Geometry: final body of the model. Coordinates: model frame, mm. Face numbers are marked on the shaded views. A direction names the side the tool comes from. Give positions to 0.01 mm unless a question says otherwise; leave off trailing zeros. Write each loop counter-clockwise with the first axis right and the second up, starting at its lowest first coordinate (ties: lowest second). Pieces come first, ordered by that corner, then holes. Notation, with made-up numbers: (3, -29.5) - (46, -29.5) arc R19 cw to (46, 0.5) - close; hole circle Ø1 at (19.25, 48). An arc over 180 degrees is marked (long way). Return JSON: item names as keys, results as strings.
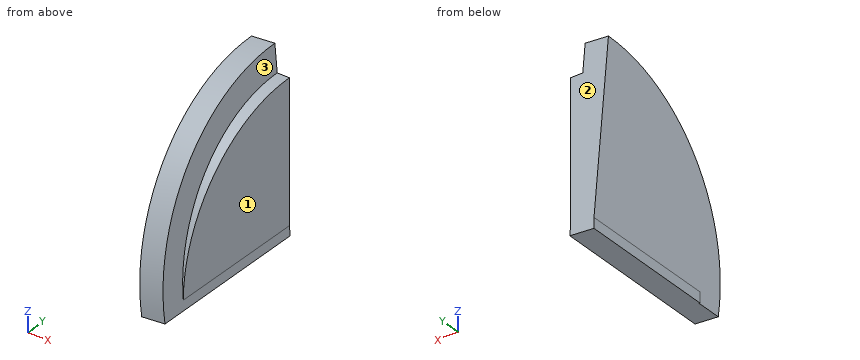
from build123d import *

# Parameters (mm, degrees)
F0_R     = 38.1
F1_DEPTH = 6.35
F4_R     = 45.0533398
F5_DEPTH = 6.35
F9_DEPTH = 50.8


with BuildPart() as f1:
    # F0 (on Right) → F1 (new body)
    with BuildSketch(Plane.YZ):
        Circle(F0_R)
    extrude(amount=F1_DEPTH)

    # F4 (on line) → F5 (join)
    with BuildSketch(Plane(origin=(0, 0, 0), x_dir=(0, 1, 0), z_dir=(0.9961946981, 0, 0.0871557427))):
        Circle(F4_R)
    extrude(amount=F5_DEPTH)

    # F8 (on offset) → F9 (cut)
    with BuildSketch(Plane(origin=(31.6291816644, 0, 2.7671948322), x_dir=(0, 1, 0), z_dir=(0.9961946981, 0, 0.0871557427))):
        Polygon((0, 54.2062856257), (0, -2.7743342798), (-63.262976706, -2.8825730551), (-87.0150923729, -54.4917583466), (75.6417736411, -57.2080314159), (68.2347118855, 54.2062856257), align=None)
    extrude(amount=-F9_DEPTH, mode=Mode.SUBTRACT)


solid = f1.part
Q1. Material intervals for probe 1 along Z at (x, y) = (1.5, -4.5); probe 2 along X at (y, z) = (-23.5, 20); probe 3 along Y at (x, z) = (4.75, 15.5), sorted ascending. Write a range as [from, to].
Answer key:
{"probe 1": "z = [-2.66, 45.13]", "probe 2": "x = [-1.75, 6.35]", "probe 3": "y = [-42.47, 0]"}
Q2. Section query B-B, the plane y = -29.5. Return the cut outline in (x, z).
Answer key:
{"outline": "(-2.97, 33.92) - (0, 0) - (0, -2.84) - (6.57, -2.26) - (6.35, 0.28) - (6.35, 24.11) - (4.26, 24.11) - (3.36, 34.48) - close"}
Q3. Pin query (flat end, axial travel): P1, Ø1, axis at x = 3.5, z = 36, coming from the -Y side; P2, Ø1.5, axis at y = -32, z = 13.5, coming from the -X side; P3, Ø10, axis at y = -37, z = 39.5, coming from the -X side; P4, Ø1.4, axis at y = -17.5, z = -2, coming from the -X side. Return the tip coordinate at first contact, or that it passes through.
Answer key:
{"P1": "stops at y = -28.2", "P2": "stops at x = -1.25", "P3": "passes through", "P4": "stops at x = 0"}
Q4. Section query C-C, the plane y = -39.5. Return the cut outline in (x, z), plus the area to 3 significant figures.
Answer key:
{"outline": "(-1.89, 21.59) - (0.25, -2.83) - (6.57, -2.28) - (4.44, 22.14) - close", "area": "156 mm^2"}
Q5. Section query A-A, the plane y = -9. Return the cut outline in (x, z).
Answer key:
{"outline": "(-3.85, 43.98) - (0, 0) - (0, -2.8) - (6.57, -2.23) - (6.35, 0.28) - (6.35, 37.02) - (3.14, 37.02) - (2.48, 44.53) - close"}
Q6. Set-up query: the marked faces 1, 2 and 3. Return all of +Z, -Z, +X, -X, +Y, -Y with unobstructed straight access to the full face (end or side cutting, diameter ignored); none if empty.
Answer key:
{"face 1": "+Z, +X, +Y, -Y", "face 2": "+Z, -Z, +X, -X, +Y", "face 3": "+Z, +X, -Y"}
